For this review, take the finished solid that the model builds, in its own axes (mm). A direction names the side the tool comes from. Coordinates: 2 decimals unless noted, no trailing zeros. Loops run counter-clockwise (first coordinate to the right, second up) from the corner with the lowest first, then second, coordinate; pieces in that order, holes last. Notation, with made-up numbers: (20.25, -15.5) - (25.25, -15.5) arc R18 cw to (25.25, 5.5) - close; hole circle Ø7 at (-37, 0.25). An arc over 180 degrees is marked (long way). Use one line per item in the form item = value. Start each with the question number.
1. To check wall thickness, follow probe 1 along Z at (x, y) = (21.15, 44.65); probe 2 along X at (y, z) = (9, 16); probe 3 along X at (y, z) = (41, -23). State the ranges of each line that lie inside material, in increasing order.
2. Add section C-C on x = -15.5. Give the boundary of the cut face in (y, z), and give its area (3 significant figures).
3. Machinability: for faces 4 (the face through (49.6, 23.07, -7.17)), 5 (the face through (56, 22, -21.4)), 6 (the face through (-41, 5, -1)), which of the approach directions +Z, -Z, +X, -X, +Y, -Y give a long, thin tool a straight path to every point of the face, cutting with its end or side? Answer none if there is none.
4. Add section B-B on z = -34. Count the separate pieces of the cut face and the enclosed holes in it, and give its area (3 significant figures).
5. For pin 1 Ø2.5 at (x, z) = (21.15, -21.95) entering from -Y; pin 2 Ø3 at (y, z) = (31, -33) entering from -X; pin 3 Ø15 at (x, z) = (66.5, -30.4) entering from -Y; pin 4 Ø2 at (x, y) = (40, 31.5) entering from -Z, all flat-tipped, find the tip position at first contact; note any pin that passes through.
6. Add section A-A on y = 31. Give the boundary of the cut face in (x, z), and give its area (3 significant figures).
7. Draft analysis for pull direction X (two halves, no side actions). For faces 1 (the face through (57, 44, -29)), 2 (the face through (15, 26, 1)), 3 (the face through (95, 23, 1)), state which applies: +X half, -X half, draft (parallel to the pull), parting line (faces both ways), or undercut.
```python
from build123d import *

# Parameters (mm, degrees)
SKETCH1_W                  = 190
SKETCH1_H                  = 80
BOSS_EXTRUDE1_DEPTH        = 5
SKETCH3_W                  = 80
SKETCH3_H                  = 80
BOSS_EXTRUDE2_DEPTH        = 42
SKETCH5_R                  = 6.5
CUT_EXTRUDE2_DEPTH         = 48
CUT_EXTRUDE3_DEPTH         = 44
SKETCH7_R                  = 3.5
CUT_EXTRUDE4_DEPTH         = 48
SKETCH8_R                  = 9.75
CUT_EXTRUDE5_DEPTH         = 48
SKETCH4_R                  = 1.55
CUT_EXTRUDE1_DEPTH         = 48
SKETCH9_R                  = 3.5
CUT_EXTRUDE6_DEPTH         = 44
SKETCH10_R                 = 10
CUT_EXTRUDE7_DEPTH         = 45.5
M3_TAPPED_HOLE1_AT_2_COUNT = 2
M3_TAPPED_HOLE1_AT_2_PITCH = 35
M3_TAPPED_HOLE1_AT_3_COUNT = 2
M3_TAPPED_HOLE1_AT_3_PITCH = 70
M3_TAPPED_HOLE2_D          = 2.5
M3_TAPPED_HOLE2_DEPTH      = 7.5
M3_TAPPED_HOLE2_TIP        = 0.751075774
M3_TAPPED_HOLE3_D          = 2.5
M3_TAPPED_HOLE3_DEPTH      = 7.5
M3_TAPPED_HOLE3_TIP        = 0.751075774
CUT_EXTRUDE8_DEPTH         = 45.5
FILLET1_R                  = 5
SKETCH_1_W                 = 68.9
SKETCH_1_H                 = 9.6
CUT_EXTRUDE_1_DEPTH        = 44


with BuildPart() as part:
    # Sketch1 → Boss-Extrude1 (new body)
    with BuildSketch(Plane(origin=(0, 0, 0), x_dir=(1, 0, 0), z_dir=(0, 1, 0))):
        Rectangle(SKETCH1_W, SKETCH1_H)
    extrude(amount=BOSS_EXTRUDE1_DEPTH)

    # Sketch3 → Boss-Extrude2 (add)
    with BuildSketch(Plane(origin=(0, 5, 0), x_dir=(1, 0, 0), z_dir=(0, 1, 0))):
        with Locations((55, 0)):
            Rectangle(SKETCH3_W, SKETCH3_H)
    extrude(amount=BOSS_EXTRUDE2_DEPTH)

    # Sketch5 → Cut-Extrude2 (cut, through all)
    with BuildSketch(Plane.XZ):
        with Locations((31.4, -30.4)):
            Circle(SKETCH5_R)
        with Locations((47.2, -30.4)):
            Circle(SKETCH5_R)
        with Locations((66.5, -30.4)):
            Circle(SKETCH5_R)
        with Locations((82.3, -30.4)):
            Circle(SKETCH5_R)
    extrude(amount=-CUT_EXTRUDE2_DEPTH, mode=Mode.SUBTRACT)

    # Sketch6 → Cut-Extrude3 (cut)
    with BuildSketch(Plane.XZ):
        with BuildLine():
            Line((31.4, -21.4), (82.3, -21.4))
            ThreePointArc((82.3, -21.4), (91.3, -30.4), (82.3, -39.4))
            Line((82.3, -39.4), (31.4, -39.4))
            ThreePointArc((31.4, -39.4), (22.4, -30.4), (31.4, -21.4))
        make_face()
    extrude(amount=-CUT_EXTRUDE3_DEPTH, mode=Mode.SUBTRACT)

    # Sketch7 → Cut-Extrude4 (cut, through all)
    with BuildSketch(Plane.XZ):
        with Locations((-84, 25)):
            Circle(SKETCH7_R)
        with Locations((-34, 25)):
            Circle(SKETCH7_R)
        with Locations((-84, -25)):
            Circle(SKETCH7_R)
        with Locations((-34, -25)):
            Circle(SKETCH7_R)
    extrude(amount=-CUT_EXTRUDE4_DEPTH, mode=Mode.SUBTRACT)

    # Sketch8 → Cut-Extrude5 (cut, through all)
    with BuildSketch(Plane.XZ):
        with Locations((26.1, 16.4)):
            Circle(SKETCH8_R)
    extrude(amount=-CUT_EXTRUDE5_DEPTH, mode=Mode.SUBTRACT)

    # Sketch4 → Cut-Extrude1 (cut, through all)
    with BuildSketch(Plane(origin=(0, 47, 0), x_dir=(1, 0, 0), z_dir=(0, 1, 0))):
        with Locations((21.15, 21.95)):
            Circle(SKETCH4_R)
        with Locations((88.15, 21.95)):
            Circle(SKETCH4_R)
        with Locations((21.15, -33.05)):
            Circle(SKETCH4_R)
        with Locations((88.15, -33.05)):
            Circle(SKETCH4_R)
    extrude(amount=-CUT_EXTRUDE1_DEPTH, mode=Mode.SUBTRACT)

    # Sketch9 → Cut-Extrude6 (cut)
    with BuildSketch(Plane.XZ):
        with Locations((21.15, -21.95)):
            Circle(SKETCH9_R)
        with Locations((88.15, -21.95)):
            Circle(SKETCH9_R)
        with Locations((21.15, 33.05)):
            Circle(SKETCH9_R)
        with Locations((88.15, 33.05)):
            Circle(SKETCH9_R)
    extrude(amount=-CUT_EXTRUDE6_DEPTH, mode=Mode.SUBTRACT)

    # Sketch10 → Cut-Extrude7 (cut)
    with BuildSketch(Plane.XZ):
        with Locations((26.1, 16.4)):
            Circle(SKETCH10_R)
    extrude(amount=-CUT_EXTRUDE7_DEPTH, mode=Mode.SUBTRACT)

    # Sketch15 → M3 Tapped Hole1 (revolve, cut)
    with BuildSketch(Plane(origin=(11.4, 2.5, -40), x_dir=(0, 1, 0), z_dir=(1, 0, 0))):
        Polygon((0, 0), (0, 9.251075774), (1.25, 8.5), (1.25, 0), align=None)
    m3_tapped_hole1 = revolve(axis=Axis((11.4, 2.5, -46.35), (0, 0, 1)), mode=Mode.SUBTRACT)

    # M3 Tapped Hole1 at 2: M3 Tapped Hole1 ×2
    with Locations(*[(-i * M3_TAPPED_HOLE1_AT_2_PITCH, 0, 0) for i in range(1, M3_TAPPED_HOLE1_AT_2_COUNT)]):
        add(m3_tapped_hole1, mode=Mode.SUBTRACT)

    # M3 Tapped Hole1 at 3: M3 Tapped Hole1 ×2
    with Locations(*[(-i * M3_TAPPED_HOLE1_AT_3_PITCH, 0, 0) for i in range(1, M3_TAPPED_HOLE1_AT_3_COUNT)]):
        add(m3_tapped_hole1, mode=Mode.SUBTRACT)

    # Mirror1: M3 Tapped Hole1 across plane
    add(m3_tapped_hole1.mirror(Plane.XY), mode=Mode.SUBTRACT)

    # Mirror1 copy 1 sketch → Mirror1 copy 1 (revolve, cut)
    with BuildSketch(Plane(origin=(-23.6, 2.5, 40), x_dir=(0, 1, 0), z_dir=(1, 0, 0))):
        Polygon((0, 0), (0, -9.251075774), (1.25, -8.5), (1.25, 0), align=None)
    revolve(axis=Axis((-23.6, 2.5, 46.35), (0, 0, 1)), mode=Mode.SUBTRACT)

    # Mirror1 copy 2 sketch → Mirror1 copy 2 (revolve, cut)
    with BuildSketch(Plane(origin=(-58.6, 2.5, 40), x_dir=(0, 1, 0), z_dir=(1, 0, 0))):
        Polygon((0, 0), (0, -9.251075774), (1.25, -8.5), (1.25, 0), align=None)
    revolve(axis=Axis((-58.6, 2.5, 46.35), (0, 0, 1)), mode=Mode.SUBTRACT)

    # M3 Tapped Hole2
    with Locations(Plane(origin=(32.5, 2.5, 40), x_dir=(1, 0, 0), z_dir=(0, 0, 1))):
        with Locations((0, 0), (45, 0)):
            Hole(M3_TAPPED_HOLE2_D / 2, depth=M3_TAPPED_HOLE2_DEPTH)
            with Locations((0, 0, -(M3_TAPPED_HOLE2_DEPTH + M3_TAPPED_HOLE2_TIP / 2))):  # 118° drill point
                Cone(0, M3_TAPPED_HOLE2_D / 2, M3_TAPPED_HOLE2_TIP, mode=Mode.SUBTRACT)

    # M3 Tapped Hole3
    with Locations(Plane(origin=(95, 2.5, 23.5), x_dir=(0, 0, 1), z_dir=(1, 0, 0))):
        with Locations((0, 0), (-35, 0)):
            Hole(M3_TAPPED_HOLE3_D / 2, depth=M3_TAPPED_HOLE3_DEPTH)
            with Locations((0, 0, -(M3_TAPPED_HOLE3_DEPTH + M3_TAPPED_HOLE3_TIP / 2))):  # 118° drill point
                Cone(0, M3_TAPPED_HOLE3_D / 2, M3_TAPPED_HOLE3_TIP, mode=Mode.SUBTRACT)

    # Sketch21 → Cut-Extrude8 (cut)
    with BuildSketch(Plane.XZ):
        Polygon((16.1, 16.4), (26.1, 16.4), (26.1, 26.4), (51.1, 26.4), (51.1, -8.6), (16.1, -8.6), align=None)
    extrude(amount=-CUT_EXTRUDE8_DEPTH, mode=Mode.SUBTRACT)

    # Fillet1
    fillet1_edges = [part.edges().sort_by_distance(p)[0] for p in [
        (16.1, 22.75, -8.6),
        (51.1, 22.75, 26.4),
        (51.1, 22.75, -8.6),
    ]]
    fillet(fillet1_edges, radius=FILLET1_R)

    # 草图1 → 切除-拉伸1 (cut)
    with BuildSketch(Plane.XZ):
        with Locations((56.85, -35.2)):
            Rectangle(SKETCH_1_W, SKETCH_1_H)
    extrude(amount=-CUT_EXTRUDE_1_DEPTH, mode=Mode.SUBTRACT)


solid = part.part
```
Conclusion:
q1.probe_1 = -40 to -23.5, -20.4 to -8.6, 25.09 to 31.5, 34.6 to 40
q1.probe_2 = 15 to 16.1, 51.1 to 95
q1.probe_3 = 15 to 17.81, 24.49 to 26.28, 91.49 to 95
q2.outline = (0, -40) - (5, -40) - (5, 40) - (0, 40) - close
q2.area = 400 mm^2
q3.face_4 = -Y
q3.face_5 = -Z, -Y
q3.face_6 = +Z, -Z, -X, +Y
q4.separate_pieces = 5
q4.enclosed_holes = 3
q4.area = 1,130 mm^2
q5.pin_1 = through
q5.pin_2 = 15
q5.pin_3 = 44
q5.pin_4 = -21.4
q6.outline = (15, -40) - (22.4, -40) - (22.4, -30.4) arc R9 cw to (31.4, -21.4) - (82.3, -21.4) arc R9 cw to (84.66, -21.71) arc R3.5 cw (long way) to (89.6, -25.14) arc R9 cw to (91.3, -30.4) - (91.3, -40) - (95, -40) - (95, 40) - (15, 40) - close; hole (16.1, -3.6) arc R5 ccw to (21.1, -8.6) - (46.1, -8.6) arc R5 ccw to (51.1, -3.6) - (51.1, 21.4) arc R5 ccw to (46.1, 26.4) - (26.1, 26.4) arc R10 ccw to (16.1, 16.4) - close; hole circle Ø7 at (21.15, -21.95); hole circle Ø7 at (21.15, 33.05); hole circle Ø7 at (88.15, 33.05)
q6.area = 3,820 mm^2
q7.face_1 = undercut
q7.face_2 = -X half
q7.face_3 = +X half
